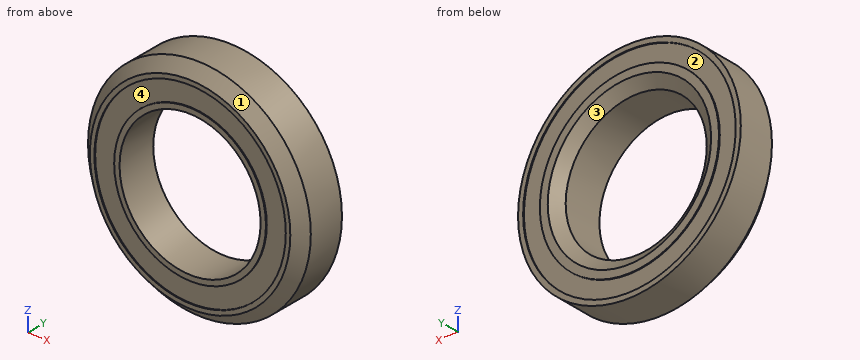
from build123d import *

# Parameters (mm, degrees)
SKETCH1_R           = 15
BOSS_EXTRUDE1_DEPTH = 6.5
SKETCH2_R           = 9.5
CUT_EXTRUDE1_DEPTH  = 7.5
CHAMFER1_SIZE       = 1.5
CHAMFER2_SIZE       = 1.5
CHAMFER2_SIZE2      = 1.089813792
SKETCH3_R           = 12.8905
SKETCH3_R_2         = 10.223184072
CUT_EXTRUDE2_DEPTH  = 0.127
SKETCH4_R           = 14.316034094
SKETCH4_R_2         = 12.065
CUT_EXTRUDE3_DEPTH  = 0.127


with BuildPart() as part:
    # Sketch1 → Boss-Extrude1 (new body)
    with BuildSketch(Plane(origin=(0, 0, 0), x_dir=(1, 0, 0), z_dir=(0, 1, 0))):
        Circle(SKETCH1_R)
    extrude(amount=BOSS_EXTRUDE1_DEPTH)

    # Sketch2 → Cut-Extrude1 (cut, through all)
    with BuildSketch(Plane(origin=(0, 6.5, 0), x_dir=(1, 0, 0), z_dir=(0, 1, 0))):
        Circle(SKETCH2_R)
    extrude(amount=-CUT_EXTRUDE1_DEPTH, mode=Mode.SUBTRACT)

    # Chamfer1
    chamfer1_edges = [part.edges().sort_by_distance(p)[0] for p in [
        (-15, 0, 0),
    ]]
    chamfer(chamfer1_edges, length=CHAMFER1_SIZE)

    # Chamfer2
    chamfer2_edges = [part.edges().sort_by_distance(p)[0] for p in [
        (-9.5, 6.5, 0),
    ]]
    chamfer2_side = [part.faces().sort_by_distance(p)[0] for p in [
        (-14.575735931, 6.5, 0),
    ]]
    chamfer(chamfer2_edges, length=CHAMFER2_SIZE, length2=CHAMFER2_SIZE2, reference=chamfer2_side[0])

    # Sketch3 → Cut-Extrude2 (cut)
    with BuildSketch(Plane.XZ):
        Circle(SKETCH3_R)
        Circle(SKETCH3_R_2, mode=Mode.SUBTRACT)
    extrude(amount=-CUT_EXTRUDE2_DEPTH, mode=Mode.SUBTRACT)

    # Sketch4 → Cut-Extrude3 (cut)
    with BuildSketch(Plane(origin=(0, 6.5, 0), x_dir=(1, 0, 0), z_dir=(0, 1, 0))):
        Circle(SKETCH4_R)
        Circle(SKETCH4_R_2, mode=Mode.SUBTRACT)
    extrude(amount=-CUT_EXTRUDE3_DEPTH, mode=Mode.SUBTRACT)


solid = part.part
Model file for the job. Use its own axes, mm. Face numbers are marked on the shaded views. A direction names the side the tool comes from. Coordinates: 2 decimals unless noted, no trailing zeros. Order: outer loops, then holes, each group sorted by start corner. A loop starts at its lowest first (then second) coordinate and runs counter-clockwise, first axis right, second up. Notation, with made-up numbers: (-5.5, -9.5) -> (22.5, -9.5) arc R15 ccw to (22.5, 9.5) -> close; hole circle Ø9 at (6.25, 28). An arc over 180 degrees is marked (long way). Return JSON: item names as keys, results as strings. Group by question number.
Item 1: Pull direction Z, two halves, no side cores. Call the marked faces 1 and 2: pulls with the +Z half, pulls with the -Z half, needs draft (parallel to the pull), parting line crosses it, or undercut.
Item 2: Saw through at C-C on y = 3.5. Write the cut outline in (x, z), then the cut area to 3 significant figures.
Item 3: Wall check: line 1 along X through (y, z) = (2.5, 0); line 2 along Z through (x, y) = (4.5, 5). Give the ranges that are in metal, low to high. Write a range as [from, to].
Item 4: Tool access for the marked faces 3 and 4: list every direction of +Z, -Z, +X, -X, +Y, -Y with a clear straight run to the whole face (end or side of a thin tool).
Item 5: Flat gauge pins, fed straight in: P1, Ø17, axis at x = 0, z = 0, coming from the +Y side; P2, Ø1, axis at y = 1, z = -5.5, coming from the +X side; P3, Ø1, axis at x = -8.5, y = 1.5, coming from the +Z side; P4, Ø2, axis at x = -9.5, y = 4.5, coming from the -Z side. Where does each tip first touch, or does it go through?
Values found:
{
 "1": {"face 1": "parting line crosses it", "face 2": "undercut"},
 "2": {"outline": "circle Ø30 at (0, 0); hole circle Ø19 at (0, 0)", "area": "423 mm2"},
 "3": {"line 1": "x = [-15, -9.5], [9.5, 15]", "line 2": "z = [-14.31, -8.37], [8.37, 14.31]"},
 "4": {"face 3": "+Y", "face 4": "-Y"},
 "5": {"P1": "passes through", "P2": "stops at x = 13.99", "P3": "stops at z = 12.69", "P4": "stops at z = -12.36"}
}
